```python
from build123d import *

# Parameters (mm, degrees)
IZIM1_W                     = 275
IZIM1_H                     = 10
Y_KSEKLIK_EKSTR_ZYON1_DEPTH = 200
IZIM2_W                     = 275
IZIM2_H                     = 10
Y_KSEKLIK_EKSTR_ZYON2_DEPTH = 10
KES_EKSTR_ZYON1_DEPTH       = 347.157478613
CUT_EXTRUDE1_REACH          = 348.157
SKETCH1_R                   = 3.5
SKETCH2_W                   = 28
SKETCH2_H                   = 21.8
CUT_EXTRUDE2_DEPTH          = 10


with BuildPart() as part:
    # Çizim1 → Yükseklik-Ekstrüzyon1 (new body)
    with BuildSketch(Plane(origin=(0, 0, 0), x_dir=(0, 0, -1), z_dir=(1, 0, 0))):
        with Locations((137.5, 5)):
            Rectangle(IZIM1_W, IZIM1_H)
    extrude(amount=Y_KSEKLIK_EKSTR_ZYON1_DEPTH)

    # Çizim2 → Yükseklik-Ekstrüzyon2 (add)
    with BuildSketch(Plane(origin=(200, 0, 0), x_dir=(0, 0, -1), z_dir=(1, 0, 0))):
        with Locations((137.5, 5)):
            Rectangle(IZIM2_W, IZIM2_H)
    extrude(amount=Y_KSEKLIK_EKSTR_ZYON2_DEPTH)

    # Çizim3 → Kes-Ekstrüzyon1 (cut, through all)
    with BuildSketch(Plane(origin=(0, 0, -275), x_dir=(-1, 0, 0), z_dir=(0, 0, -1))):
        Polygon((-210, 10), (-200, 0), (-210, 0), align=None)
    extrude(amount=-KES_EKSTR_ZYON1_DEPTH, mode=Mode.SUBTRACT)

    # Sketch1 → Cut-Extrude1 (cut, up to next)
    with BuildSketch(Plane(origin=(0, 10, 0), x_dir=(1, 0, 0), z_dir=(0, 1, 0)), mode=Mode.PRIVATE) as cut_extrude1_sk1:
        with Locations(Location((95, 176.01, 0), (0, 0, 270))):
            Circle(SKETCH1_R)
    cut_extrude1_tool1 = extrude(cut_extrude1_sk1.sketch, amount=-CUT_EXTRUDE1_REACH, mode=Mode.PRIVATE) & part.part
    # Sketch1 → Cut-Extrude1 (cut, up to next)
    with BuildSketch(Plane(origin=(0, 10, 0), x_dir=(1, 0, 0), z_dir=(0, 1, 0)), mode=Mode.PRIVATE) as cut_extrude1_sk2:
        with Locations(Location((164.5, 176.01, 0), (0, 0, 270))):
            Circle(SKETCH1_R)
    cut_extrude1_tool2 = extrude(cut_extrude1_sk2.sketch, amount=-CUT_EXTRUDE1_REACH, mode=Mode.PRIVATE) & part.part
    # Sketch1 → Cut-Extrude1 (cut, up to next)
    with BuildSketch(Plane(origin=(0, 10, 0), x_dir=(1, 0, 0), z_dir=(0, 1, 0)), mode=Mode.PRIVATE) as cut_extrude1_sk3:
        with Locations(Location((95, 112.01, 0), (0, 0, 270))):
            Circle(SKETCH1_R)
    cut_extrude1_tool3 = extrude(cut_extrude1_sk3.sketch, amount=-CUT_EXTRUDE1_REACH, mode=Mode.PRIVATE) & part.part
    # Sketch1 → Cut-Extrude1 (cut, up to next)
    with BuildSketch(Plane(origin=(0, 10, 0), x_dir=(1, 0, 0), z_dir=(0, 1, 0)), mode=Mode.PRIVATE) as cut_extrude1_sk4:
        with Locations(Location((164.5, 112.01, 0), (0, 0, 270))):
            Circle(SKETCH1_R)
    cut_extrude1_tool4 = extrude(cut_extrude1_sk4.sketch, amount=-CUT_EXTRUDE1_REACH, mode=Mode.PRIVATE) & part.part
    add(cut_extrude1_tool1.solids().sort_by_distance((95, 10, -176.01))[0], mode=Mode.SUBTRACT)
    add(cut_extrude1_tool2.solids().sort_by_distance((164.5, 10, -176.01))[0], mode=Mode.SUBTRACT)
    add(cut_extrude1_tool3.solids().sort_by_distance((95, 10, -112.01))[0], mode=Mode.SUBTRACT)
    add(cut_extrude1_tool4.solids().sort_by_distance((164.5, 10, -112.01))[0], mode=Mode.SUBTRACT)

    # Sketch2 → Cut-Extrude2 (cut)
    with BuildSketch(Plane(origin=(0, 10, 0), x_dir=(1, 0, 0), z_dir=(0, 1, 0))):
        with Locations((32.090687836, 250.029608882)):
            Rectangle(SKETCH2_W, SKETCH2_H)
    extrude(amount=-CUT_EXTRUDE2_DEPTH, mode=Mode.SUBTRACT)


solid = part.part
```
Here's how the part is built. I have some questions about the finished solid (model axes, mm). A direction names the side the tool comes from. Coordinates: 2 decimals unless noted, no trailing zeros. Order: outer loops, then holes, each group sorted by start corner. A loop starts at its lowest first (then second) coordinate and runs counter-clockwise, first axis right, second up. Notation, with made-up numbers: (-37, -7) -> (21, -7) arc R23 ccw to (21, 4) -> close; hole circle Ø3 at (51.25, 65). An arc over 180 degrees is marked (long way). Return JSON: item names as keys, results as strings.
1) If we section it at D-D on z = -30: List the corners of the cut face in (x, y) for me, plus the area to 3 significant figures.
Conclusion:
{"outline": "(0, 0) -> (200, 0) -> (210, 10) -> (0, 10) -> close", "area": "2,050 mm²"}
2) If I drill on probe 1 along Z at (x, y) = (164.5, 8.25); probe 2 along Z at (x, y) = (45, 2.25); probe 3 along X at (y, z) = (4.75, -176.01), over which ranges is the centre line in solid material (lowest first)?
Conclusion:
{"probe 1": "z = -275 to -179.51, -172.51 to -115.51, -108.51 to 0", "probe 2": "z = -275 to -260.93, -239.13 to 0", "probe 3": "x = 0 to 91.5, 98.5 to 161, 168 to 204.75"}
3) On a 3-axis mill with a long thin cutter (end or side, diameter ignored), from which of +Z, -Z, +X, -X, +Y, -Y can I reach the whole of each face in a straight line? I mean faces 4 (the flat face through (32, 5, -239.13)), 5 (the flat face through (104, 10, -136)). Say none if no direction works.
Conclusion:
{"face 4": "+Y, -Y", "face 5": "+Z, -Z, +X, -X, +Y"}
4) Thinking about a two-plate mould opening in Z: for faces 1 (the flat face through (104, 5, -275)), 2 (the flat face through (104, 5, 0)), 3 (the cylindrical face through (91.583, 5.07, -176.769)), which applies, +Z half, -Z half, draft (parallel to the pull), parting line (faces both ways), or undercut?
Conclusion:
{"face 1": "-Z half", "face 2": "+Z half", "face 3": "undercut"}
5) If we section it at B-B on x = 164.5: List the corners of the cut face in (y, z) for me, plus the area to 3 significant figures.
Conclusion:
{"outline": "(0, -275) -> (10, -275) -> (10, -179.51) -> (0, -179.51) -> close; (0, -172.51) -> (10, -172.51) -> (10, -115.51) -> (0, -115.51) -> close; (0, -108.51) -> (10, -108.51) -> (10, 0) -> (0, 0) -> close", "area": "2,610 mm²"}
6) If we section it at A-A on y = 4.5: List the corners of the cut face in (x, z) for me, plus the area to 3 significant figures.
Conclusion:
{"outline": "(0, -275) -> (204.5, -275) -> (204.5, 0) -> (0, 0) -> close; hole (18.09, -260.93) -> (46.09, -260.93) -> (46.09, -239.13) -> (18.09, -239.13) -> close; hole circle Ø7 at (95, -176.01); hole circle Ø7 at (95, -112.01); hole circle Ø7 at (164.5, -176.01); hole circle Ø7 at (164.5, -112.01)", "area": "55,500 mm²"}
7) I'm going to push flat-ended pins straight in: P1, Ø4, axis at x = 164.5, z = -112.01, coming from the -Y side; P2, Ø3, axis at y = 1.5, z = -172.5, coming from the +X side; P3, Ø3, axis at y = 5, z = -248.5, coming from the +X side; P4, Ø1, axis at y = 4, z = -96, coming from the +X side. Where does each tip first touch, or does it pass through?
Conclusion:
{"P1": "passes through", "P2": "stops at x = 203", "P3": "stops at x = 206.5", "P4": "stops at x = 204.5"}
8) If we section it at C-C on z = -112.01: List the corners of the cut face in (x, y) for me.
Conclusion:
{"outline": "(0, 0) -> (91.5, 0) -> (91.5, 10) -> (0, 10) -> close; (98.5, 0) -> (161, 0) -> (161, 10) -> (98.5, 10) -> close; (168, 0) -> (200, 0) -> (210, 10) -> (168, 10) -> close"}
